Design review of the part built by this model. Coordinates are the model's own, in mm. Coordinates: 2 decimals unless noted, no trailing zeros. Write each loop counter-clockwise with the first axis right and the second up, starting at its lowest first coordinate (ties: lowest second). Pieces come first, ordered by that corner, then holes. Notation, with made-up numbers: (29.5, 82.25) - (57.5, 82.25) arc R5 cw to (57.5, 88.25) - close; hole circle Ø5 at (13.5, 45). An arc over 180 degrees is marked (long way). Answer as CSV lines item,"result". Start each with the question number.
Q1. Mouldability with a two-part tool opening along X and no side actions: class faces 1 (the face through (12.65, -0.04, -4.48)), 2 (the face through (6.5, -3.5, 0)), 3 (the face through (-13.887, 10.648, -2.746)), 4 (the face through (-12.7, -0.3, -4.5)) as pulls with the +X half, pulls with the -X half, needs draft (parallel to the pull), parting line crosses it, or undercut.
Q2. Clearance check with flat-ended pins moving along their axes: pin 1 (2 mm diameter, centred on y = -9, z = -2.5, fed in from -X); pin 2 (5 mm diameter, centred on x = 8, y = -0.5, fed in from -Z). State where each tip first meets the part, or that it passes through.
Q3. For line 1 along Z through (x, y) = (5.5, 12); line 2 along X through (y, z) = (-8.5, -0.25); line 3 along X through (y, z) = (6, -0.5), list the stretches that pass through material, from the lowest coordinate up. Write a range as [from, to].
Q4. We need section A-A (z = -4.75). Write out the cut boundary in (x, y).
from build123d import *

# Parameters (mm, degrees)
F2_SIZE  = 2.5
F3_R     = 0.9
F4_DEPTH = 3


with BuildPart() as f1:
    # F0 (on Front) → F1 (revolve)
    with BuildSketch(Plane.XZ):
        with BuildLine():
            Line((17.5, 0), (7.064701, 0))
            ThreePointArc((7.064701, 0), (8.141347, -1.412911), (8.939239, -3))
            Line((8.939239, -3), (17.5, -3))
            Line((17.5, -3), (17.5, 0))
        make_face()
    revolve(axis=Axis((0, 0, -4.75), (0, 0, -1)))

    # F2
    f2_edges = [f1.edges().sort_by_distance(p)[0] for p in [
        (-17.5, 0, 0),
    ]]
    chamfer(f2_edges, length=F2_SIZE)

    # F3 (on face) → F4 (join)
    with BuildSketch(Plane(origin=(0, 0, -3), x_dir=(1, 0, 0), z_dir=(0, 0, -1))):
        with Locations((-13.55, 0)):
            Circle(F3_R)
        with Locations((13.55, 0)):
            Circle(F3_R)
    extrude(amount=F4_DEPTH)


solid = f1.part
Results list:
1,face 1,"undercut"
1,face 2,"needs draft"
1,face 3,"parting line crosses it"
1,face 4,"undercut"
2,pin 1,"stops at x = -15.56"
2,pin 2,"stops at z = -3"
3,line 1,"z = [-3, 0]"
3,line 2,"x = [-12.66, 12.66]"
3,line 3,"x = [-14.29, -4.49], [4.49, 14.29]"
4,outline,"circle Ø1.8 at (-13.55, 0); circle Ø1.8 at (13.55, 0)"
